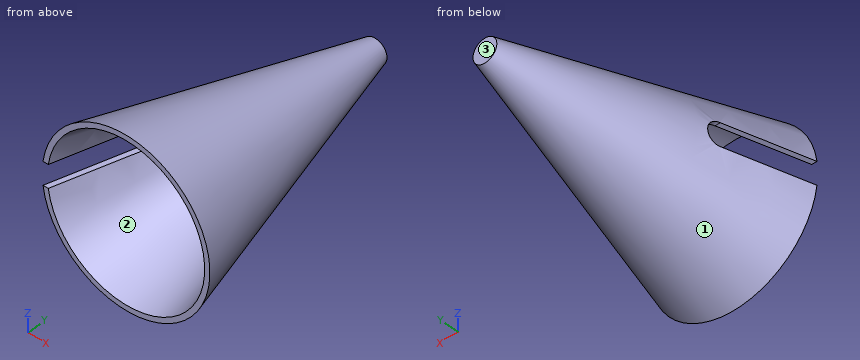
Autodesk Inventor part; units mm, degrees
ref_plane "YZ Plane" through (0, 0, 0) normal (1, 0, 0) x (0, 1, 0)
ref_plane "XZ Plane" through (0, 0, 0) normal (0, 1, 0) x (-1, 0, 0)
ref_plane "XY Plane" through (0, 0, 0) normal (0, 0, 1) x (1, 0, 0)
sketch "Sketch1" plane through (0, 0, 0) normal (0, 0, 1) x (1, 0, 0)
  line L0 (0, 0) -> (0, 41.4782)
  line L1 (0, 41.4782) -> (-1.27, 41.4782)
  line L2 (-1.27, 41.4782) -> (-12.3841, 0)
  line L3 (-12.3841, 0) -> (0, 0)
  line L4 (0, -8.2956) -> (0, 49.7738)
  dimension "d0" = 1.27
  dimension "d1" = 75
  dimension "d2" = 41.4782
revolve "Revolution1" add sketch "Sketch1" angle 360 about axis through (0, -10, 0) along (0, 1, 0)
shell "Shell1" thickness 0.7937 outward yes removed faces 1 at (4.0081, 0, 0.9879)
sketch "Sketch2" plane through (0, 0, 0) normal (1, 0, 0) x (0, 1, 0)
  line L0 (0, 0) -> (12.7, 0) construction
  line L1 (0, -1.7996) -> (12.7, -1.7996)
  line L2 (12.7, 1.7996) -> (0, 1.7996)
  arc A0 (0, 1.7996) -> (0, -1.7996) centre (0, 0) ccw
  arc A1 (12.7, -1.7996) -> (12.7, 1.7996) centre (12.7, 0) ccw
  line L3 (0, -13.2058) -> (0, 13.2058)
  point P0 (6.35, 0)
  dimension "d7" = 1.7996
  dimension "d8" = 6.35
extrude "Extrusion1" cut sketch "Sketch2" against normal through all contours L3 L2 A1 L1
properties part number "CC-01" material "Steel, Galvanized"
Build history of the part. All positions in model axes, mm. Face numbers are marked on the shaded views. Give positions to 0.01 mm unless a question says otherwise; leave off trailing zeros. Order: outer loops, then holes, each group sorted by start corner. A loop starts at its lowest first (then second) coordinate and runs counter-clockwise, first axis right, second up. Notation, with made-up numbers: M 27.25,26.5 L 67.25,26.5 A9 cw 67.25,32.5 Z; hole C -22,60.5 d9. An arc over 180 degrees is marked long. Put each result on its own line as item: value.
Item 1: Probe line 1 (Z direction, x = 7.75, y = 7); line 2 (Z direction, x = 0.75, y = 35); line 3 (X direction, y = 29, z = -3.5). List the from-to ranges inside material, lowest first. Write a range as [from, to].
From the geometry:
line 1: z = [-8.26, -7.1], [7.1, 8.26]
line 2: z = [-3.75, -2.91], [2.91, 3.75]
line 3: x = [-4.16, -3.01], [3.01, 4.16]
Item 2: Slice it at A-A, the plane x = 0. Write the cut outline in (y, z), plus the area to 3 significant figures.
From the geometry:
outline: M 0,-13.21 L 42.27,-1.88 L 42.27,1.88 L 0,13.21 L 0,12.38 L 41.48,1.27 L 41.48,-1.27 L 0,-12.38 Z
area: 71.3 mm2
Item 3: Slice it at C-C, the plane y = 30. Write the cut outline in (x, z).
From the geometry:
outline: C 0,0 d10.33; hole C 0,0 d8.69
Item 4: Slice it at B-B, the plane z = 0. Write the cut outline in (x, y), plus the area to 3 significant figures.
From the geometry:
outline: M -9.32,14.5 L -8.5,14.5 L -1.27,41.48 L 1.27,41.48 L 12.38,0 L 13.21,0 L 1.88,42.27 L -1.88,42.27 Z
area: 59.4 mm2
Item 5: Slice it at D-D, the plane y = 22. Write the cut outline in (x, z), plus the area to 3 significant figures.
From the geometry:
outline: C 0,0 d14.62; hole C 0,0 d12.98
area: 35.6 mm2
Item 6: Flat gauge pins, fed straight in: pin 1 Ø1 at (x, y) = (-5.5, 29) entering from -Z; pin 2 Ø3.5 at (x, y) = (-11.5, 9) entering from -Z; pin 3 Ø1 at (x, y) = (-5.5, 22) entering from -Z. Where does each tip first touch, or does it go through?
From the geometry:
pin 1: stops at z = -2.18
pin 2: stops at z = -4.79
pin 3: stops at z = -5.37
Item 7: Two-plate mould, pull along X, no slides. Class the marked faces 1, 2 and 3: +X half, -X half, draft (parallel to the pull), parting line (faces both ways), or undercut.
From the geometry:
face 1: parting line
face 2: undercut
face 3: draft
